```python
from build123d import *

# Parameters (mm, degrees)
SKETCH1_W           = 13.7
SKETCH1_H           = 15.7
BOSS_EXTRUDE1_DEPTH = 30
SKETCH2_R           = 5
BOSS_EXTRUDE2_DEPTH = 24
SKETCH3_R           = 10
BOSS_EXTRUDE3_DEPTH = 26.2
SKETCH4_R           = 5
BOSS_EXTRUDE4_DEPTH = 3
SKETCH5_R           = 3.15
BOSS_EXTRUDE5_DEPTH = 18
SKETCH8_R           = 1.5
CUT_EXTRUDE1_DEPTH  = 2


with BuildPart() as part:
    # Sketch1 → Boss-Extrude1 (new body)
    with BuildSketch(Plane(origin=(0, 0, 0), x_dir=(1, 0, 0), z_dir=(0, 1, 0))):
        Rectangle(SKETCH1_W, SKETCH1_H)
    extrude(amount=BOSS_EXTRUDE1_DEPTH)

    # Sketch2 → Boss-Extrude2 (add)
    with BuildSketch(Plane.XZ):
        Circle(SKETCH2_R)
    extrude(amount=BOSS_EXTRUDE2_DEPTH)

    # Sketch3 → Boss-Extrude3 (add)
    with BuildSketch(Plane.XZ.offset(24)):
        Circle(SKETCH3_R)
    extrude(amount=BOSS_EXTRUDE3_DEPTH)

    # Sketch4 → Boss-Extrude4 (add)
    with BuildSketch(Plane.XZ.offset(50.2)):
        Circle(SKETCH4_R)
    extrude(amount=BOSS_EXTRUDE4_DEPTH)

    # Sketch5 → Boss-Extrude5 (add)
    with BuildSketch(Plane(origin=(0, 30, 0), x_dir=(1, 0, 0), z_dir=(0, 1, 0))):
        Circle(SKETCH5_R)
    extrude(amount=BOSS_EXTRUDE5_DEPTH)

    # Sketch8 → Cut-Extrude1 (cut)
    with BuildSketch(Plane(origin=(0, 0, -7.85), x_dir=(-1, 0, 0), z_dir=(0, 0, -1))):
        with Locations((0, 8)):
            Circle(SKETCH8_R)
        with Locations((0, 22.8)):
            Circle(SKETCH8_R)
    extrude(amount=-CUT_EXTRUDE1_DEPTH, mode=Mode.SUBTRACT)


solid = part.part
```
Verification items for the finished model (mm, model axes). A direction names the side the tool comes from. Round coordinates to 2 decimals unless told otherwise and drop trailing zeros. Write each loop counter-clockwise with the first axis right and the second up, starting at its lowest first coordinate (ties: lowest second). Pieces come first, ordered by that corner, then holes. Notation, with made-up numbers: (55, 83.25) -> (97, 83.25) arc R23 cw to (97, 95.25) -> close; hole circle Ø9 at (30, 82). An arc over 180 degrees is marked (long way). Write each question's results on one line, items separated by ' | '. Start each with the question number.
1. Cross-section at A-A (y = 8). Enter the section's corners in (x, z), then the cut area to 3 significant figures.
2. Depth check by flat-ended pin: P1, Ø3.5, axis at x = 0, y = 22.8, coming from the -Z side; P2, Ø12, axis at x = -5.5, z = 5, coming from the -Y side; P3, Ø12, axis at y = -11.5, z = -0.5, coming from the -X side; P4, Ø1.8, axis at x = 0, y = 8, coming from the -Z side. Enter the tip coordinate at first touch or a pass-through.
3. Cross-section at B-B (x = 0). Enter the section's corners in (y, z).
4. Cross-section at D-D (x = 8.75). Enter the section's corners in (y, z), then the cut area to 3 significant figures.
5. Material ranges on probe 1 along Y at (x, z) = (0, -6.3); probe 2 along Y at (x, z) = (-4.5, -6.75); probe 3 along Y at (x, z) = (1.5, -3.75), recorded low to high. Write a range as from..to.
6. Cross-section at C-C (z = -4). Enter the section's corners in (x, y).
7. Set-up check for faces 1 (the cylindrical face through (-1.08, -51.68, -4.88)), 2 (the flat face through (-5, 0, -2)), 3 (the cylindrical face through (0.325, 21.336, -6.864)), 4 (the flat face through (-6.85, 15, 0)), 5 (the flat face through (6.85, 15, 0)): record each of +Z, -Z, +X, -X, +Y, -Y from which the full face is reachable in a straight line by a thin tool's end or side.
Solutions:
1) outline: (-6.85, -7.85) -> (-1.5, -7.85) -> (-1.5, -5.85) -> (1.5, -5.85) -> (1.5, -7.85) -> (6.85, -7.85) -> (6.85, 7.85) -> (-6.85, 7.85) -> close | area: 209 mm2
2) P1: stops at z = -7.85 | P2: stops at y = -53.2 | P3: stops at x = -5 | P4: stops at z = -5.85
3) outline: (-53.2, -5) -> (-50.2, -5) -> (-50.2, -10) -> (-24, -10) -> (-24, -5) -> (0, -5) -> (0, -7.85) -> (6.5, -7.85) -> (6.5, -5.85) -> (9.5, -5.85) -> (9.5, -7.85) -> (21.3, -7.85) -> (21.3, -5.85) -> (24.3, -5.85) -> (24.3, -7.85) -> (30, -7.85) -> (30, -3.15) -> (48, -3.15) -> (48, 3.15) -> (30, 3.15) -> (30, 7.85) -> (0, 7.85) -> (0, 5) -> (-24, 5) -> (-24, 10) -> (-50.2, 10) -> (-50.2, 5) -> (-53.2, 5) -> close
4) outline: (-50.2, -4.84) -> (-24, -4.84) -> (-24, 4.84) -> (-50.2, 4.84) -> close | area: 254 mm2
5) probe 1: y = -50.2..-24, 0..6.5, 9.5..21.3, 24.3..30 | probe 2: y = -50.2..-24, 0..30 | probe 3: y = -53.2..30
6) outline: (-9.17, -50.2) -> (-3, -50.2) -> (-3, -53.2) -> (3, -53.2) -> (3, -50.2) -> (9.17, -50.2) -> (9.17, -24) -> (3, -24) -> (3, 0) -> (6.85, 0) -> (6.85, 30) -> (-6.85, 30) -> (-6.85, 0) -> (-3, 0) -> (-3, -24) -> (-9.17, -24) -> close
7) face 1: -Y | face 2: none | face 3: -Z | face 4: +Z, -Z, -X, +Y | face 5: +Z, -Z, +X, +Y
